Here's how the part is built. I have some questions about the finished solid (model axes, mm). Face numbers are marked on the shaded views. A direction names the side the tool comes from. Round coordinates to 2 decimals unless told otherwise and drop trailing zeros. Loops run counter-clockwise (first coordinate to the right, second up) from the corner with the lowest first, then second, coordinate; pieces in that order, holes last. Notation, with made-up numbers: (-38, -12) - (-19, -12) arc R25 cw to (-19, 27) - close; hole circle Ø2 at (32, 83). An arc over 180 degrees is marked (long way). Return JSON: item names as keys, results as strings. Group by question number.
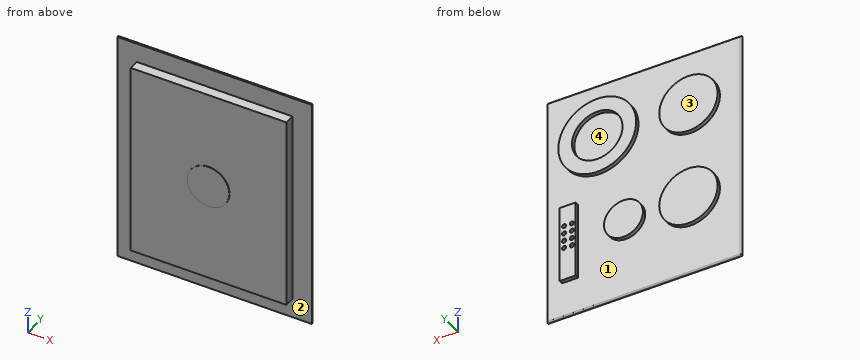
```python
from build123d import *

# Parameters (mm, degrees)
SKETCH1_W           = 500
SKETCH1_H           = 600
BOSS_EXTRUDE1_DEPTH = 6
FILLET1_R           = 3
SKETCH3_W           = 400
SKETCH3_H           = 500
BOSS_EXTRUDE2_DEPTH = 26
SKETCH2_R           = 75
SKETCH2_R_2         = 50
SKETCH2_R_3         = 100
SKETCH2_R_4         = 65
SKETCH2_W           = 41.104529262
SKETCH2_H           = 200
SKETCH2_R_5         = 5.399416509
BOSS_EXTRUDE3_DEPTH = 10
SKETCH4_R           = 53.966181138
BOSS_EXTRUDE4_DEPTH = 1


with BuildPart() as part:
    # Sketch1 → Boss-Extrude1 (new body)
    with BuildSketch(Plane(origin=(0, 0, 0), x_dir=(1, 0, 0), z_dir=(0, 1, 0))):
        with Locations((250, 300)):
            Rectangle(SKETCH1_W, SKETCH1_H)
    extrude(amount=BOSS_EXTRUDE1_DEPTH)

    # Fillet1
    fillet1_edges = [part.edges().sort_by_distance(p)[0] for p in [
        (500, 6, -300),
        (250, 6, -600),
        (0, 6, -300),
        (250, 6, 0),
    ]]
    fillet(fillet1_edges, radius=FILLET1_R)

    # Sketch3 → Boss-Extrude2 (add)
    with BuildSketch(Plane.XZ):
        with Locations((250, -300)):
            Rectangle(SKETCH3_W, SKETCH3_H)
    extrude(amount=BOSS_EXTRUDE2_DEPTH)

    # Sketch2 → Boss-Extrude3 (add)
    with BuildSketch(Plane(origin=(0, 6, 0), x_dir=(1, 0, 0), z_dir=(0, 1, 0))):
        with Locations((130.089337479, 397)):
            Circle(SKETCH2_R)
        with Locations((297, 397)):
            Circle(SKETCH2_R_2)
        with Locations((130.089337479, 143.740125968)):
            Circle(SKETCH2_R)
        with Locations((364.330089408, 143.740125968)):
            Circle(SKETCH2_R_3)
        with Locations((364.330089408, 143.740125968)):
            Circle(SKETCH2_R_4, mode=Mode.SUBTRACT)
        with Locations((440.198970532, 407)):
            Rectangle(SKETCH2_W, SKETCH2_H)
        with Locations((449.543954361, 420.752043301)):
            Circle(SKETCH2_R_5, mode=Mode.SUBTRACT)
        with Locations((429.543954361, 420.752043301)):
            Circle(SKETCH2_R_5, mode=Mode.SUBTRACT)
        with Locations((429.543954361, 400.752043301)):
            Circle(SKETCH2_R_5, mode=Mode.SUBTRACT)
        with Locations((429.543954361, 380.752043301)):
            Circle(SKETCH2_R_5, mode=Mode.SUBTRACT)
        with Locations((429.543954361, 360.752043301)):
            Circle(SKETCH2_R_5, mode=Mode.SUBTRACT)
        with Locations((449.543954361, 400.752043301)):
            Circle(SKETCH2_R_5, mode=Mode.SUBTRACT)
        with Locations((449.543954361, 380.752043301)):
            Circle(SKETCH2_R_5, mode=Mode.SUBTRACT)
        with Locations((449.543954361, 360.752043301)):
            Circle(SKETCH2_R_5, mode=Mode.SUBTRACT)
    extrude(amount=BOSS_EXTRUDE3_DEPTH)

    # Sketch4 → Boss-Extrude4 (add)
    with BuildSketch(Plane.XZ.offset(26)):
        with Locations((250, -300)):
            Circle(SKETCH4_R)
    extrude(amount=BOSS_EXTRUDE4_DEPTH)


solid = part.part
```
Q1. Imagine slicing it at C-C, the plane x = 409. List the corners of the cut face in (y, z) for me, and give its area (3 significant figures).
Q2. If we mould it in two halves opening along X, with no side actions, what happens to the marked faces 1 and 2? For each: +X half, -X half, draft (parallel to the pull), parting line (faces both ways), or undercut.
Q3. Imagine slicing it at A-A, the plane x = 62.5. List the corners of the cut face in (y, z) for me, and give its area (3 significant figures).
Q4. Please list where these lines run through material, in increasing order: line 1 (X direction, y = -13, z = -129.5); line 2 (Z direction, x = 426, y = -13.5); line 3 (Y direction, x = 365, z = -322).
Q5. Will these pins go through, and if not, where does the flat tip stop? pin 1 Ø5 at (x, y) = (436.5, 11.5) entering from -Z; pin 2 Ø5.5 at (x, z) = (429, -359) entering from +Y; pin 3 Ø5 at (x, z) = (67.5, -462) entering from -Y; pin 4 Ø5 at (y, z) = (3.5, -205) entering from +X.
Q6. Imagine slicing it at D-D, the plane x = 283.5. List the corners of the cut face in (y, z) for me, and give its area (3 significant figures).
Q7. Imagine slicing it at B-B, the plane y = -17. List the corners of the cut face in (x, z) for me, and give its area (3 significant figures).
Q8. For the marked faces 3 and 4, which set-ups out of +Z, -Z, +X, -X, +Y, -Y let a thin tool reach every point of the face, with its end or its side?
Output values:
{
 "1": {"outline": "(-26, -550) - (0, -550) - (0, -600) - (3, -600) arc R3 ccw to (6, -597) - (6, -233.21) - (16, -233.21) - (16, -190.96) - (6, -190.96) - (6, -96.52) - (16, -96.52) - (16, -54.27) - (6, -54.27) - (6, -3) arc R3 ccw to (3, 0) - (0, 0) - (0, -50) - (-26, -50) - close", "area": "17,400 mm^2"},
 "2": {"face 1": "undercut", "face 2": "draft"},
 "3": {"outline": "(-26, -550) - (0, -550) - (0, -600) - (3, -600) arc R3 ccw to (6, -597) - (6, -429.51) - (16, -429.51) - (16, -364.49) - (6, -364.49) - (6, -176.25) - (16, -176.25) - (16, -111.23) - (6, -111.23) - (6, -3) arc R3 ccw to (3, 0) - (0, 0) - (0, -50) - (-26, -50) - close", "area": "17,900 mm^2"},
 "4": {"line 1": "x = 50 to 450", "line 2": "z = -550 to -50", "line 3": "y = -26 to 6"},
 "5": {"pin 1": "stops at z = -507", "pin 2": "stops at y = 6", "pin 3": "stops at y = -26", "pin 4": "stops at x = 500"},
 "6": {"outline": "(-27, -342.31) - (-26, -342.31) - (-26, -550) - (0, -550) - (0, -600) - (3, -600) arc R3 ccw to (6, -597) - (6, -445.14) - (16, -445.14) - (16, -348.86) - (6, -348.86) - (6, -202.62) - (16, -202.62) - (16, -84.86) - (6, -84.86) - (6, -3) arc R3 ccw to (3, 0) - (0, 0) - (0, -50) - (-26, -50) - (-26, -257.69) - (-27, -257.69) - close", "area": "18,800 mm^2"},
 "7": {"outline": "(50, -550) - (450, -550) - (450, -50) - (50, -50) - close", "area": "200,000 mm^2"},
 "8": {"face 3": "+Z, -Z, +X, -X, +Y", "face 4": "+Y"}
}
